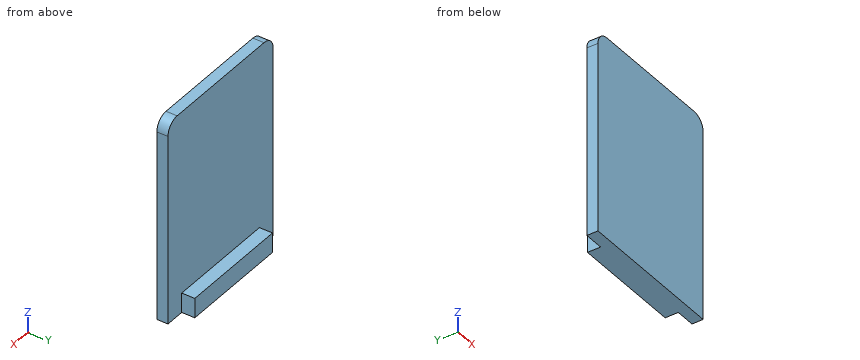
Autodesk Inventor part; units mm, degrees
ref_plane "YZ Plane" through (0, 0, 0) normal (1, 0, 0) x (0, 1, 0)
ref_plane "XZ Plane" through (0, 0, 0) normal (0, 1, 0) x (-1, 0, 0)
ref_plane "XY Plane" through (0, 0, 0) normal (0, 0, 1) x (1, 0, 0)
sketch "스케치1" plane through (0, 0, 0) normal (0, 1, 0) x (-1, 0, 0)
  line L0 (0, 0) -> (11.5, 0)
  line L1 (11.5, 0) -> (11.5, -15.5)
  line L2 (11.5, -15.5) -> (0, -15.5)
  line L3 (0, -15.5) -> (0, 0)
  dimension "d0" = 11.5
  dimension "d1" = 15.5
extrude "돌출1" add sketch "스케치1" along normal blind 0.85
fillet "모깎기1" radius 1 2 edges at (0, 0.425, 0) (-11.5, 0.425, 0)
sketch "스케치2" plane through (0, 0.85, 0) normal (0, 1, 0) x (1, 0, 0)
  line L0 (0, 1) -> (0, 15.5)
  line L1 (0, 15.5) -> (-11.5, 15.5)
  line L2 (-1.5, 15.5) -> (-10, 15.5)
  line L3 (-10, 15.5) -> (-10, 14)
  line L4 (-10, 14) -> (-1.5, 14)
  line L5 (-1.5, 14) -> (-1.5, 15.5)
  line L6 (-11.5, 15.5) -> (-11.5, 1)
  point P0 (0, 0)
  dimension "d5" = 8.5
  dimension "d6" = 1.5
  dimension "d7" = 1.5
  dimension "d13" = 1.5
extrude "돌출2" add sketch "스케치2" along normal blind 1
equation "\"d7\" = d13"
properties part number "_3D 인쇄"
Build history of the part. All positions in model axes, mm. Round coordinates to 2 decimals unless told otherwise and drop trailing zeros. Loops run counter-clockwise (first coordinate to the right, second up) from the corner with the lowest first, then second, coordinate; pieces in that order, holes last.
Item 1: Saw through at A-A (y = 1.1). List the corners of the cut face in (x, z).
Item 2: Saw through at C-C (x = -8.5). List the corners of the cut face in (y, z), then the cut area to 3 significant figures.
Item 3: Pin check, flat tips, straight feed: P1, Ø1, axis at x = -3, z = -10, coming from the -Y side; P2, Ø3, axis at x = -9, z = -4.5, coming from the +Y side; P3, Ø1.1, axis at y = 1.5, z = -15, coming from the +X side. Stop position of each tip, or through.
Item 4: Saw through at B-B (z = -2). List the corners of the cut face in (x, y).
Item 5: Drill centre lines: line 1 along Z through (x, y) = (-8, 1.7); line 2 along Y through (x, z) = (-7.25, -12). Where is each one in solid material? Low to high.
Worked answers:
1. outline: (-10, -15.5) - (-1.5, -15.5) - (-1.5, -14) - (-10, -14) - close
2. outline: (0, -15.5) - (1.85, -15.5) - (1.85, -14) - (0.85, -14) - (0.85, 0) - (0, 0) - close
2. area: 14.7 mm2
3. P1: stops at y = 0
3. P2: stops at y = 0.85
3. P3: stops at x = -1.5
4. outline: (-11.5, 0) - (0, 0) - (0, 0.85) - (-11.5, 0.85) - close
5. line 1: z = -15.5 to -14
5. line 2: y = 0 to 0.85
